Part print with two shaded views. Sizes in mm from the minimum x, y, z corner. A direction names the side the tool comes from. Coordinates: 2 decimals unless noted, no trailing zeros. Loops run counter-clockwise (first coordinate to the right, second up) from the corner with the lowest first, then second, coordinate; pieces in that order, holes last. Notation, with made-up numbers: (27.25, -32.5) -> (40.25, -32.5) arc R22 ccw to (40.25, -22.5) -> close; hole circle Ø2 at (64, 86). An arc over 180 degrees is marked (long way). Return JSON: item names as keys, results as strings. Group by question number.
(1) Flat gauge pins, fed straight in: pin 1 Ø1.5 at (x, z) = (49, 18.5) entering from -Y; pin 2 Ø0.9 at (x, z) = (42.5, 11) entering from -Y; pin 3 Ø0.8 at (y, z) = (1.5, 8.5) entering from +X; pin 4 Ø2 at (x, z) = (15.5, 18) entering from +Y. Where does each tip first touch, or does it go through?
(2) Tool access for the marked faces 1 and 2: list every direction of +Z, -Z, +X, -X, +Y, -Y with a clear straight run to the whole face (end or side of a thin tool).
(3) Saw through at A-A on x = 29. Write the cut outline in (y, z).
(4) Saw through at D-D on y = 7. Write the cut outline in (x, z).
(5) Saw through at C-C on y = 1.5. Write the cut outline in (x, z).
(6) Probe L1, parallel to Z at x = 11, y = 7.25; L2, parallel to X at y = 3.5, z = 28; L3, parallel to Y at x = 48.5, z = 23. List the from-to ranges inside material, lowest first.
(7) Mould opens along Z. For the marked faces 3, 4 and 5 say: pulls with the +Z half, pulls with the -Z half, needs draft (parallel to the pull), parting line crosses it, or undercut.
(8) Saw through at B-B on z = 3. Write the cut outline in (x, y).
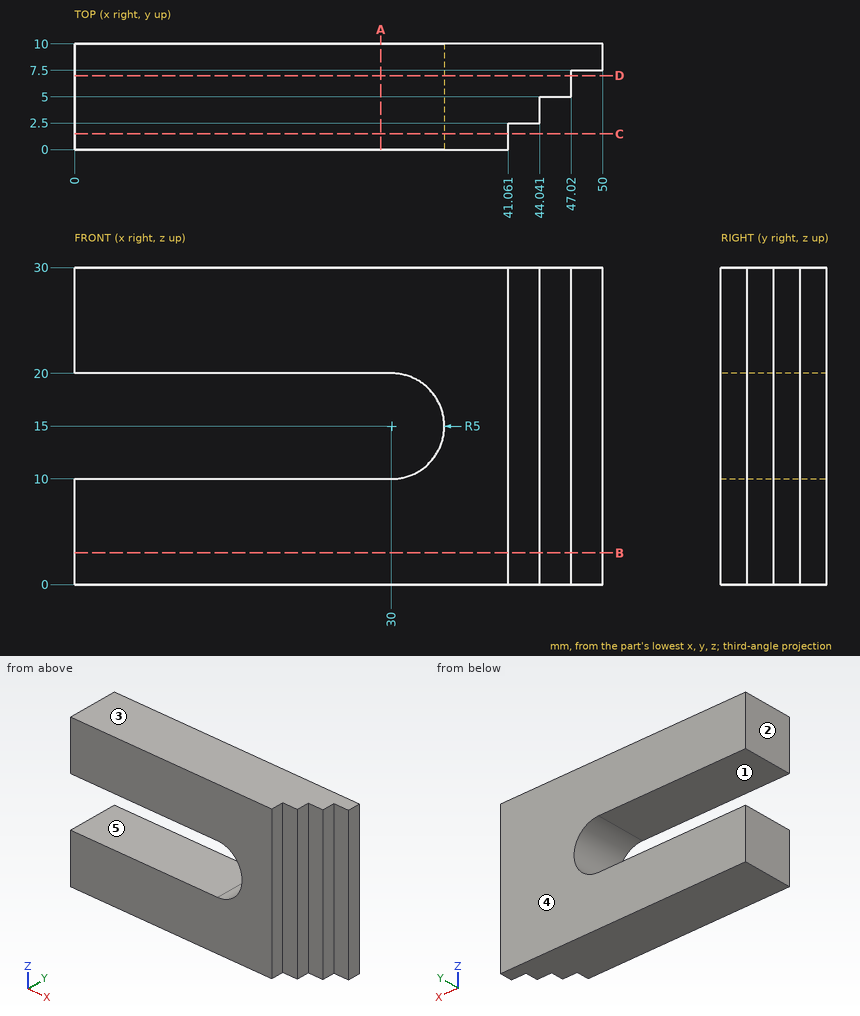
Geometry results:
{
 "1": {"pin 1": "y = 7.5", "pin 2": "y = 2.5", "pin 3": "x = 41.06", "pin 4": "through"},
 "2": {"face 1": "-X, +Y, -Y", "face 2": "+Z, -Z, -X, +Y, -Y"},
 "3": {"outline": "(0, 0) -> (10, 0) -> (10, 10) -> (0, 10) -> close; (0, 20) -> (10, 20) -> (10, 30) -> (0, 30) -> close"},
 "4": {"outline": "(0, 0) -> (47.02, 0) -> (47.02, 30) -> (0, 30) -> (0, 20) -> (30, 20) arc R5 cw to (30, 10) -> (0, 10) -> close"},
 "5": {"outline": "(0, 0) -> (41.06, 0) -> (41.06, 30) -> (0, 30) -> (0, 20) -> (30, 20) arc R5 cw to (30, 10) -> (0, 10) -> close"},
 "6": {"L1": "0 to 10, 20 to 30", "L2": "0 to 44.04", "L3": "7.5 to 10"},
 "7": {"face 3": "pulls with the +Z half", "face 4": "needs draft", "face 5": "undercut"},
 "8": {"outline": "(0, 0) -> (41.06, 0) -> (41.06, 2.5) -> (44.04, 2.5) -> (44.04, 5) -> (47.02, 5) -> (47.02, 7.5) -> (50, 7.5) -> (50, 10) -> (0, 10) -> close"}
}
